```python
from build123d import *

# Parameters (mm, degrees)
SKETCH1_W           = 6
SKETCH1_H           = 2
BOSS_EXTRUDE1_DEPTH = 3
FILLET1_R           = 5
BOSS_EXTRUDE2_DEPTH = 3
CUT_EXTRUDE1_REACH  = 167.708
SKETCH3_R           = 1.325
SKETCH3_W           = 20
SKETCH3_H           = 5
FILLET2_R           = 2
FILLET3_R           = 2


with BuildPart() as part:
    # Sketch1 → Boss-Extrude1 (new body)
    with BuildSketch(Plane(origin=(0, 0, 0), x_dir=(1, 0, 0), z_dir=(0, 1, 0))):
        Polygon((-153, 5), (-165, 5), (-165, 2.5), (-157.5, -5), (157.5, -5), (165, 2.5), (165, 5), (153, 5), (147, 5), (-147, 5), align=None)
        with Locations((-150, 6)):
            Rectangle(SKETCH1_W, SKETCH1_H)
        with Locations((150, 6)):
            Rectangle(SKETCH1_W, SKETCH1_H)
    extrude(amount=BOSS_EXTRUDE1_DEPTH)

    # Fillet1
    fillet1_edges = [part.edges().sort_by_distance(p)[0] for p in [
        (157.5, 1.5, 5),
        (-157.5, 1.5, 5),
        (-165, 1.5, -2.5),
        (165, 1.5, -2.5),
    ]]
    fillet(fillet1_edges, radius=FILLET1_R)

    # Sketch2 → Boss-Extrude2 (add)
    with BuildSketch(Plane(origin=(0, 3, 0), x_dir=(1, 0, 0), z_dir=(0, 1, 0))):
        with BuildLine():
            Line((-38.653805922, -15), (-30.951902961, -7.298097039))
            ThreePointArc((-30.951902961, -7.298097039), (-34.493721155, -8.002608481), (-36.5, -5))
            Line((-36.5, -5), (-63.5, -5))
            ThreePointArc((-63.5, -5), (-65.506278845, -8.002608481), (-69.048097039, -7.298097039))
            Line((-69.048097039, -7.298097039), (-61.346194078, -15))
            Line((-61.346194078, -15), (-38.653805922, -15))
        make_face()
        with BuildLine():
            Line((-65.425, -5), (-63.5, -5))
            ThreePointArc((-63.5, -5), (-66.75, -1.75), (-70, -5))
            Line((-70, -5), (-68.075, -5))
            ThreePointArc((-68.075, -5), (-66.75, -3.675), (-65.425, -5))
        make_face()
        with BuildLine():
            ThreePointArc((-69.048097039, -7.298097039), (-65.506278845, -8.002608481), (-63.5, -5))
            Line((-63.5, -5), (-65.425, -5))
            ThreePointArc((-65.425, -5), (-66.75, -6.325), (-68.075, -5))
            Line((-68.075, -5), (-70, -5))
            ThreePointArc((-70, -5), (-69.752608481, -6.243721155), (-69.048097039, -7.298097039))
        make_face()
        with BuildLine():
            ThreePointArc((-30.951902961, -7.298097039), (-30.247391519, -6.243721155), (-30, -5))
            Line((-30, -5), (-31.925, -5))
            ThreePointArc((-31.925, -5), (-33.25, -6.325), (-34.575, -5))
            Line((-34.575, -5), (-36.5, -5))
            ThreePointArc((-36.5, -5), (-34.493721155, -8.002608481), (-30.951902961, -7.298097039))
        make_face()
        with BuildLine():
            Line((-31.925, -5), (-30, -5))
            ThreePointArc((-30, -5), (-33.25, -1.75), (-36.5, -5))
            Line((-36.5, -5), (-34.575, -5))
            ThreePointArc((-34.575, -5), (-33.25, -3.675), (-31.925, -5))
        make_face()
        with BuildLine():
            Line((61.346194078, -15), (69.048097039, -7.298097039))
            ThreePointArc((69.048097039, -7.298097039), (65.506278845, -8.002608481), (63.5, -5))
            Line((63.5, -5), (36.5, -5))
            ThreePointArc((36.5, -5), (34.493721155, -8.002608481), (30.951902961, -7.298097039))
            Line((30.951902961, -7.298097039), (38.653805922, -15))
            Line((38.653805922, -15), (61.346194078, -15))
        make_face()
        with BuildLine():
            Line((31.925, -5), (30, -5))
            ThreePointArc((30, -4.999999997), (30.247391519, -6.243721154), (30.951902961, -7.298097039))
            ThreePointArc((30.951902961, -7.298097039), (34.493721155, -8.002608481), (36.5, -5))
            Line((36.5, -5), (34.575, -5))
            ThreePointArc((34.575, -5), (33.25, -6.325), (31.925, -5))
        make_face()
        with BuildLine():
            ThreePointArc((36.5, -5), (33.250000002, -1.75), (30, -4.999999997))
            Line((30, -5), (31.925, -5))
            ThreePointArc((31.925, -5), (33.25, -3.675), (34.575, -5))
            Line((34.575, -5), (36.5, -5))
        make_face()
        with BuildLine():
            Line((68.075, -5), (70, -5))
            ThreePointArc((70, -5), (66.75, -1.75), (63.5, -5))
            Line((63.5, -5), (65.425, -5))
            ThreePointArc((65.425, -5), (66.75, -3.675), (68.075, -5))
        make_face()
        with BuildLine():
            ThreePointArc((69.048097039, -7.298097039), (69.752608481, -6.243721155), (70, -5))
            Line((70, -5), (68.075, -5))
            ThreePointArc((68.075, -5), (66.75, -6.325), (65.425, -5))
            Line((65.425, -5), (63.5, -5))
            ThreePointArc((63.5, -5), (65.506278845, -8.002608481), (69.048097039, -7.298097039))
        make_face()
    extrude(amount=-BOSS_EXTRUDE2_DEPTH)

    # Sketch3 → Cut-Extrude1 (cut, up to next)
    with BuildSketch(Plane(origin=(0, 3, 0), x_dir=(1, 0, 0), z_dir=(0, 1, 0)), mode=Mode.PRIVATE) as cut_extrude1_sk1:
        with Locations(Location((-66.75, -5, 0), (0, 0, 270))):
            Circle(SKETCH3_R)
    cut_extrude1_tool1 = extrude(cut_extrude1_sk1.sketch, amount=-CUT_EXTRUDE1_REACH, mode=Mode.PRIVATE) & part.part
    # Sketch3 → Cut-Extrude1 (cut, up to next)
    with BuildSketch(Plane(origin=(0, 3, 0), x_dir=(1, 0, 0), z_dir=(0, 1, 0)), mode=Mode.PRIVATE) as cut_extrude1_sk2:
        with Locations(Location((-33.25, -5, 0), (0, 0, 270))):
            Circle(SKETCH3_R)
    cut_extrude1_tool2 = extrude(cut_extrude1_sk2.sketch, amount=-CUT_EXTRUDE1_REACH, mode=Mode.PRIVATE) & part.part
    # Sketch3 → Cut-Extrude1 (cut, up to next)
    with BuildSketch(Plane(origin=(0, 3, 0), x_dir=(1, 0, 0), z_dir=(0, 1, 0)), mode=Mode.PRIVATE) as cut_extrude1_sk3:
        with Locations(Location((33.25, -5, 0), (0, 0, 270))):
            Circle(SKETCH3_R)
    cut_extrude1_tool3 = extrude(cut_extrude1_sk3.sketch, amount=-CUT_EXTRUDE1_REACH, mode=Mode.PRIVATE) & part.part
    # Sketch3 → Cut-Extrude1 (cut, up to next)
    with BuildSketch(Plane(origin=(0, 3, 0), x_dir=(1, 0, 0), z_dir=(0, 1, 0)), mode=Mode.PRIVATE) as cut_extrude1_sk4:
        with Locations(Location((66.75, -5, 0), (0, 0, 270))):
            Circle(SKETCH3_R)
    cut_extrude1_tool4 = extrude(cut_extrude1_sk4.sketch, amount=-CUT_EXTRUDE1_REACH, mode=Mode.PRIVATE) & part.part
    # Sketch3 → Cut-Extrude1 (cut, up to next)
    with BuildSketch(Plane(origin=(0, 3, 0), x_dir=(1, 0, 0), z_dir=(0, 1, 0)), mode=Mode.PRIVATE) as cut_extrude1_sk5:
        with Locations((0, -2.5)):
            Rectangle(SKETCH3_W, SKETCH3_H)
    cut_extrude1_tool5 = extrude(cut_extrude1_sk5.sketch, amount=-CUT_EXTRUDE1_REACH, mode=Mode.PRIVATE) & part.part
    # Sketch3 → Cut-Extrude1 (cut, up to next)
    with BuildSketch(Plane(origin=(0, 3, 0), x_dir=(1, 0, 0), z_dir=(0, 1, 0)), mode=Mode.PRIVATE) as cut_extrude1_sk6:
        with BuildLine():
            Line((13, -1.25), (13, -3.75))
            ThreePointArc((13, -3.75), (12.926776695, -3.926776695), (12.75, -4))
            Line((12.75, -4), (11.75, -4))
            ThreePointArc((11.75, -4), (11.573223305, -3.926776695), (11.5, -3.75))
            Line((11.5, -3.75), (11.5, -1.25))
            ThreePointArc((11.5, -1.25), (11.573223305, -1.073223305), (11.75, -1))
            Line((11.75, -1), (12.75, -1))
            ThreePointArc((12.75, -1), (12.926776695, -1.073223305), (13, -1.25))
        make_face()
    cut_extrude1_tool6 = extrude(cut_extrude1_sk6.sketch, amount=-CUT_EXTRUDE1_REACH, mode=Mode.PRIVATE) & part.part
    # Sketch3 → Cut-Extrude1 (cut, up to next)
    with BuildSketch(Plane(origin=(0, 3, 0), x_dir=(1, 0, 0), z_dir=(0, 1, 0)), mode=Mode.PRIVATE) as cut_extrude1_sk7:
        with BuildLine():
            Line((-12.75, -1), (-11.75, -1))
            ThreePointArc((-11.75, -1), (-11.573223305, -1.073223305), (-11.5, -1.25))
            Line((-11.5, -1.25), (-11.5, -3.75))
            ThreePointArc((-11.5, -3.75), (-11.573223305, -3.926776695), (-11.75, -4))
            Line((-11.75, -4), (-12.75, -4))
            ThreePointArc((-12.75, -4), (-12.926776695, -3.926776695), (-13, -3.75))
            Line((-13, -3.75), (-13, -1.25))
            ThreePointArc((-13, -1.25), (-12.926776695, -1.073223305), (-12.75, -1))
        make_face()
    cut_extrude1_tool7 = extrude(cut_extrude1_sk7.sketch, amount=-CUT_EXTRUDE1_REACH, mode=Mode.PRIVATE) & part.part
    add(cut_extrude1_tool1.solids().sort_by_distance((-66.75, 3, 5))[0], mode=Mode.SUBTRACT)
    add(cut_extrude1_tool2.solids().sort_by_distance((-33.25, 3, 5))[0], mode=Mode.SUBTRACT)
    add(cut_extrude1_tool3.solids().sort_by_distance((33.25, 3, 5))[0], mode=Mode.SUBTRACT)
    add(cut_extrude1_tool4.solids().sort_by_distance((66.75, 3, 5))[0], mode=Mode.SUBTRACT)
    add(cut_extrude1_tool5.solids().sort_by_distance((0, 3, 2.5))[0], mode=Mode.SUBTRACT)
    add(cut_extrude1_tool6.solids().sort_by_distance((12.25, 3, 2.5))[0], mode=Mode.SUBTRACT)
    add(cut_extrude1_tool7.solids().sort_by_distance((-12.25, 3, 2.5))[0], mode=Mode.SUBTRACT)

    # Fillet2
    fillet2_edges = [part.edges().sort_by_distance(p)[0] for p in [
        (-30, 1.5, 5),
        (-70, 1.5, 5),
        (-61.346194078, 1.5, 15),
        (-38.653805922, 1.5, 15),
        (61.346194078, 1.5, 15),
        (38.653805922, 1.5, 15),
        (30, 1.5, 5),
        (70, 1.5, 5),
    ]]
    fillet(fillet2_edges, radius=FILLET2_R)

    # Fillet3
    fillet3_edges = [part.edges().sort_by_distance(p)[0] for p in [
        (10, 1.5, 0),
        (10, 1.5, 5),
        (-10, 1.5, 5),
        (-10, 1.5, 0),
    ]]
    fillet(fillet3_edges, radius=FILLET3_R)


solid = part.part
```
Verification items for the finished model (mm, model axes). A direction names the side the tool comes from. Give positions to 0.01 mm unless a question says otherwise; leave off trailing zeros. Order: outer loops, then holes, each group sorted by start corner. A loop starts at its lowest first (then second) coordinate and runs counter-clockwise, first axis right, second up. Notation, with made-up numbers: M -2,32.25 L 53,32.25 A19 ccw 53,63.25 Z; hole C 53,64 d4. An arc over 180 degrees is marked long. Answer in a Markdown table with one row per item. Add a question column.
Item 1: Section check A-A, the plane y = 0.6. State how many separate pieces and enclosed holes the cut face has, and give its area (3 significant figures).
Item 2: Scan lines: probe 1 along X at (y, z) = (1.7, 2.25); probe 2 along X at (y, z) = (1.8, 1.5); probe 3 along Z at (x, y) = (56.5, 1.35). Record each from-to range of solid material in increasing order. Write a range as from..to.
Item 3: Gauge pin test, flat ends, axial feed: pin 1 (0.6 mm diameter, centred on y = 1.5, z = -6, fed in from +X); pin 2 (1.5 mm diameter, centred on x = 23, y = 1, fed in from -Z); pin 3 (1.5 mm diameter, centred on x = 11.5, y = 1.5, fed in from +Z). Record the tip position at first contact, or that the pin passes through.
Item 4: Tool access check on faces 1 (the flat face through (-34.56, 1.521, 10.906)), 2 (the flat face through (-2, 0, -1)). Record the directions out of +Z, -Z, +X, -X, +Y, -Y that give a thin tool (end or side, any length) a straight path to the whole face; none if there is none.
Item 5: Section check B-B, the plane x = 16.5. Enter the section's corners in (y, z), and give its area (3 significant figures).
Filled sheet:
| question | item | result |
|---|---|---|
| 1 | separate pieces | 1 |
| 1 | enclosed holes | 6 |
| 1 | area | 3,790 mm^2 |
| 2 | probe 1 | x = -160.25..-13, -11.5..-10, 10..11.5, 13..160.25 |
| 2 | probe 2 | x = -161..-13, -11.5..-9.94, 9.94..11.5, 13..161 |
| 2 | probe 3 | z = -5..15 |
| 3 | pin 1 | stops at x = 153 |
| 3 | pin 2 | stops at z = -5 |
| 3 | pin 3 | stops at z = 5 |
| 4 | face 1 | +Z, +Y, -Y |
| 4 | face 2 | +Z, -Z, +X, -X, -Y |
| 5 | outline | M 0,-5 L 3,-5 L 3,5 L 0,5 Z |
| 5 | area | 30.0 mm^2 |
